```python
from build123d import *

# Parameters (mm, degrees)
BOSS_EXTRUDE1_DEPTH = 30
SKETCH1_3_W         = 35
SKETCH1_3_H         = 35
SKETCH1_3_R         = 7.5
BOSS_EXTRUDE2_DEPTH = 10


with BuildPart() as part:
    # Sketch1 → Boss-Extrude1 (new body)
    with BuildSketch(Plane.XY):
        Polygon((10, 0), (10, 25), (30, 25), (30, 0), (40, 0), (40, 35), (0, 35), (0, 0), align=None)
    extrude(amount=BOSS_EXTRUDE1_DEPTH)

    # Sketch1_3 → Boss-Extrude2 (add)
    # profile 1 of 2: a face of its own
    with BuildSketch(Plane.XY):
        Polygon((0, 0), (10, 0), (10, 25), (30, 25), (30, 0), (40, 0), (40, 35), (0, 35), align=None)
    # profile 2 of 2: a face of its own
    with BuildSketch(Plane.XY):
        with Locations((57.5, 17.5)):
            Rectangle(SKETCH1_3_W, SKETCH1_3_H)
        with Locations((57.5, 17.5)):
            Circle(SKETCH1_3_R, mode=Mode.SUBTRACT)
    extrude(amount=BOSS_EXTRUDE2_DEPTH)


solid = part.part
```
Geometry: final body of the model. Coordinates: model frame, mm. A direction names the side the tool comes from. Round coordinates to 2 decimals unless told otherwise and drop trailing zeros. Write each loop counter-clockwise with the first axis right and the second up, starting at its lowest first coordinate (ties: lowest second). Pieces come first, ordered by that corner, then holes. Notation, with made-up numbers: (83, 11) -> (127, 11) arc R23 ccw to (127, 48) -> close; hole circle Ø8 at (71, -6.75). An arc over 180 degrees is marked (long way). Use CSV: the item, a comma, the result in double quotes. Start each with the question number.
Q1. Section B-B (z = 13). Return loops of the section in (x, y).
Q2. Pull-direction query (Y, two-part tool) for faces 4 (the face through (20, 25, 15)), 5 (the face through (52, 22.6, 4.9)), 6 (the face through (30, 35, 11)), 7 (the face through (10, 12, 15)); classes: pulls with the +Y half, pulls with the -Y half, needs draft (parallel to the pull), parting line crosses it, or undercut.
Q3. Line query: L1, parallel to X at y = 3, z = 28.25; L2, parallel to Y at x = 57.5, z = 7.75; L3, parallel to Z at x = 42, y = 8.5. Output: solid intervals per line, ascending.
Q4. Section A-A (y = 23.5). Return loops of the section in (x, z), plus the area to 3 significant figures.
Q5. Reachability of faces 1 (the face through (20, 26, 30)), 2 (the face through (30, 13, 15)), 3 (the face through (40, 17, 20)) from +Z, -Z, +X, -X, +Y, -Y: full face, straight path, thin tool, end or side. Return the list, or none.
Q6. Section D-D (y = 7.5). Return loops of the section in (x, z), plus the area to 3 significant figures.
Q7. First-contact query: pin 1 Ø6 at (x, z) = (21.5, 10) entering from -Y; pin 2 Ø1 at (y, z) = (30, 24) entering from +X; pin 3 Ø17.5 at (x, y) = (56.5, 23) entering from +Z; pin 4 Ø13.5 at (x, y) = (57.5, 17.5) entering from +Z. Flat tips, straight axial feed; report the tip coordinate or a pass-through.
Q8. Section C-C (x = 57.5). Return loops of the section in (y, z), plus the area to 3 significant figures.
Result sheet:
1,outline,"(0, 0) -> (10, 0) -> (10, 25) -> (30, 25) -> (30, 0) -> (40, 0) -> (40, 35) -> (0, 35) -> close"
2,face 4,"pulls with the -Y half"
2,face 5,"undercut"
2,face 6,"pulls with the +Y half"
2,face 7,"needs draft"
3,L1,"0 to 10, 30 to 40"
3,L2,"0 to 10, 25 to 35"
3,L3,"0 to 10"
4,outline,"(0, 0) -> (10, 0) -> (10, 30) -> (0, 30) -> close; (30, 0) -> (53, 0) -> (53, 10) -> (40, 10) -> (40, 30) -> (30, 30) -> close; (62, 0) -> (75, 0) -> (75, 10) -> (62, 10) -> close"
4,area,"860 mm²"
5,face 1,"+Z, +X, -X, +Y, -Y"
5,face 2,"+Z, -Z, -Y"
5,face 3,"+Z, +X, +Y, -Y"
6,outline,"(0, 0) -> (10, 0) -> (10, 30) -> (0, 30) -> close; (30, 0) -> (75, 0) -> (75, 10) -> (40, 10) -> (40, 30) -> (30, 30) -> close"
6,area,"950 mm²"
7,pin 1,"y = 25"
7,pin 2,"x = 40"
7,pin 3,"z = 10"
7,pin 4,"through"
8,outline,"(0, 0) -> (10, 0) -> (10, 10) -> (0, 10) -> close; (25, 0) -> (35, 0) -> (35, 10) -> (25, 10) -> close"
8,area,"200 mm²"
